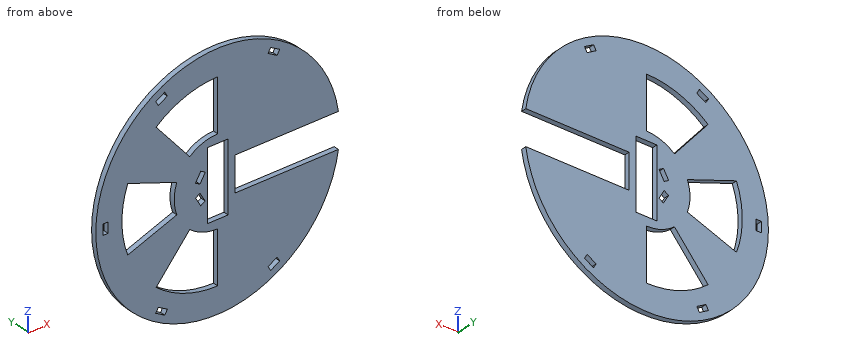
Autodesk Inventor part; units mm, degrees
ref_plane "YZ Plane" through (0, 0, 0) normal (1, 0, 0) x (0, 1, 0)
ref_plane "XZ Plane" through (0, 0, 0) normal (0, 1, 0) x (-1, 0, 0)
ref_plane "XY Plane" through (0, 0, 0) normal (0, 0, 1) x (1, 0, 0)
sketch "草圖1" plane through (0, 0, 0) normal (0, 1, 0) x (-1, 0, 0)
  circle A0 centre (0, 0) radius 70
  circle A1 centre (0, 0) radius 25
  line L0 (-70, 10) -> (-10, 10)
  line L1 (-10, 10) -> (-10, -10)
  line L2 (-10, -10) -> (-70, -10)
  line L3 (-70, -10) -> (-70, 10)
  line L4 (0, 0) -> (0, -55)
  line L5 (0, 0) -> (35.3533, -42.1324)
  arc A2 (0, -55) -> (35.3533, -42.1324) centre (0, 0) ccw
  line L6 (0, 0) -> (51.6831, -18.8111)
  line L7 (0, 0) -> (51.6831, 18.8111)
  arc A3 (51.6831, -18.8111) -> (51.6831, 18.8111) centre (0, 0) ccw
  line L8 (0, 0) -> (35.3533, 42.1324)
  line L9 (0, 0) -> (0, 55)
  arc A4 (35.3533, 42.1324) -> (0, 55) centre (0, 0) ccw
  line L10 (-9.3, -13.3795) -> (-36.7, -13.3795)
  line L11 (-36.7, -13.3795) -> (-36.7, -69.3795)
  line L12 (-36.7, -69.3795) -> (-9.3, -69.3795)
  line L13 (-9.3, -69.3795) -> (-9.3, -13.3795)
  line L14 (-7.8, -20.3795) -> (-10.8, -20.3795)
  line L15 (-10.8, -20.3795) -> (-10.8, -27.3795)
  line L16 (-10.8, -27.3795) -> (-7.8, -27.3795)
  line L17 (-7.8, -27.3795) -> (-7.8, -20.3795)
  line L18 (-7.8, -55.3795) -> (-10.8, -55.3795)
  line L19 (-10.8, -55.3795) -> (-10.8, -62.3795)
  line L20 (-10.8, -62.3795) -> (-7.8, -62.3795)
  line L21 (-7.8, -62.3795) -> (-7.8, -55.3795)
  line L22 (-35.2, -20.3795) -> (-38.2, -20.3795)
  line L23 (-38.2, -20.3795) -> (-38.2, -27.3795)
  line L24 (-38.2, -27.3795) -> (-35.2, -27.3795)
  line L25 (-35.2, -27.3795) -> (-35.2, -20.3795)
  line L26 (-35.2, -48.3795) -> (-38.2, -48.3795)
  line L27 (-38.2, -48.3795) -> (-38.2, -55.3795)
  line L28 (-38.2, -55.3795) -> (-35.2, -55.3795)
  line L29 (-35.2, -55.3795) -> (-35.2, -48.3795)
  circle A5 centre (0, 0) radius 2
  line L30 (-1.5, 1.3229) -> (-1.5, -1.3229)
  point P0 (-23, -13.3795)
  point P1 (-9.3, -20.3795)
  point P2 (-9.3, -62.3795)
  point P3 (-36.7, -20.3795)
  point P4 (-36.7, -48.3795)
  point P5 (16.0697, -19.1511)
  point P6 (0, -25)
  point P7 (-69.282, 10)
  point P8 (-69.282, -10)
  point P9 (16.0697, 19.1511)
  point P10 (0, 25)
  point P11 (23.4923, -8.5505)
  point P12 (23.4923, 8.5505)
  point P13 (-70, 0)
  dimension "d0" = 140
  dimension "d1" = 50
  dimension "d2" = 20
  dimension "d3" = 60
  dimension "d4" = 55
  dimension "d5" = 40
  dimension "d6" = 55
  dimension "d9" = 140
  dimension "d11" = 13
  dimension "d12" = 27.4
  dimension "d13" = 56
  dimension "d14" = 7
  dimension "d15" = 3
  dimension "d16" = 7
  dimension "d17" = 7
  dimension "d18" = 3
  dimension "d19" = 7
  dimension "d20" = 7
  dimension "d21" = 3
  dimension "d22" = 7
  dimension "d23" = 7
  dimension "d24" = 3
  dimension "d25" = 21
  dimension "d28" = 4
  dimension "d29" = 1.5
extrude "擠出1" add sketch "草圖1" along normal blind 3 contours L13 L20 L21 L18 L16 L17 A1 L4 A2 L5 L6 A3 L7 L8 A4 L9 L0 A0 | A0 L11 L28 L29 L26 L24 L25 L22 L10 A1 L15 L16 L13 L18 L19 L20 | A0 L2 A1 L10 L11 L22 L23 L24 L26 L27 L28 | L20 L19 L18 L13 | L13 L18 L21 L20 | L28 L27 L26 L11 | L11 L26 L29 L28 | A1 L9 A5 L4 L17 L14 L13 L10 L2 L1 L0 | L16 L15 A1 L13 | L13 A1 L17 L16 | A1 L8 A5 L9 | L10 L13 L14 L15 A1 | L24 L23 L22 L11 | L11 L22 L25 L24 | L13 L14 L17 A1 | A1 L15 L14 L13 | A1 L7 A5 L8 | A1 L6 A5 L7 | L30 A5 | L4 A5 L5 A1 | A5 L6 A1 L5
sketch "草圖2" plane through (0, 3, 0) normal (0, 1, 0) x (1, 0, 0)
  line L0 (-3, 13) -> (3, 13)
  line L1 (3, 13) -> (3, 10)
  line L2 (3, 10) -> (-3, 10)
  line L3 (-3, 10) -> (-3, 13)
  line L4 (-12.7583, 3.9019) -> (-9.7583, 9.0981)
  line L5 (-9.7583, 9.0981) -> (-7.1603, 7.5981)
  line L6 (-7.1603, 7.5981) -> (-10.1603, 2.4019)
  line L7 (-10.1603, 2.4019) -> (-12.7583, 3.9019)
  line L8 (-9.7583, -9.0981) -> (-12.7583, -3.9019)
  line L9 (-12.7583, -3.9019) -> (-10.1603, -2.4019)
  line L10 (-10.1603, -2.4019) -> (-7.1603, -7.5981)
  line L11 (-7.1603, -7.5981) -> (-9.7583, -9.0981)
  line L12 (3, -13) -> (-3, -13)
  line L13 (-3, -13) -> (-3, -10)
  line L14 (-3, -10) -> (3, -10)
  line L15 (3, -10) -> (3, -13)
  line L16 (-66, 3) -> (-63, 3)
  line L17 (-63, 3) -> (-63, -3)
  line L18 (-63, -3) -> (-66, -3)
  line L19 (-66, -3) -> (-66, 3)
  line L20 (-34.0981, -53.0596) -> (-28.9019, -56.0596)
  line L21 (-28.9019, -56.0596) -> (-30.4019, -58.6577)
  line L22 (-30.4019, -58.6577) -> (-35.5981, -55.6577)
  line L23 (-35.5981, -55.6577) -> (-34.0981, -53.0596)
  line L24 (28.9019, -56.0596) -> (34.0981, -53.0596)
  line L25 (34.0981, -53.0596) -> (35.5981, -55.6577)
  line L26 (35.5981, -55.6577) -> (30.4019, -58.6577)
  line L27 (30.4019, -58.6577) -> (28.9019, -56.0596)
  line L28 (63, -3) -> (63, 3)
  line L29 (63, 3) -> (66, 3)
  line L30 (66, 3) -> (66, -3)
  line L31 (66, -3) -> (63, -3)
  line L32 (34.0981, 53.0596) -> (28.9019, 56.0596)
  line L33 (28.9019, 56.0596) -> (30.4019, 58.6577)
  line L34 (30.4019, 58.6577) -> (35.5981, 55.6577)
  line L35 (35.5981, 55.6577) -> (34.0981, 53.0596)
  line L36 (-28.9019, 56.0596) -> (-34.0981, 53.0596)
  line L37 (-34.0981, 53.0596) -> (-35.5981, 55.6577)
  line L38 (-35.5981, 55.6577) -> (-30.4019, 58.6577)
  line L39 (-30.4019, 58.6577) -> (-28.9019, 56.0596)
  point P0 (0, 0)
  point P1 (0, 10)
  point P2 (-8.6603, 5)
  point P3 (-8.6603, -5)
  point P4 (0, -10)
  point P5 (-63, 0)
  point P6 (-31.5, -54.5596)
  point P7 (31.5, -54.5596)
  point P8 (63, 0)
  point P9 (31.5, 54.5596)
  point P10 (-31.5, 54.5596)
  dimension "d30" = 3
  dimension "d31" = 6
  dimension "d32" = 10
  dimension "d35" = 180
  dimension "d46" = 3
  dimension "d47" = 6
  dimension "d48" = 63
  dimension "d51" = 360
extrude "擠出2" cut sketch "草圖2" against normal through all contours L0 L1 L2 L3 | L4 L5 L6 L7 | L8 L9 L10 L11 | L12 L13 L14 L15 | L16 L17 L18 L19 | L20 L21 L22 L23 | L24 L25 L26 L27 | L32 L33 L34 L35 | L36 L37 L38 L39
sketch "草圖3" plane through (0, 3, 0) normal (0, 1, 0) x (1, 0, 0)
  circle A0 centre (0, 0) radius 6
  line L0 (-6, 20) -> (6, 20)
  line L1 (6, 20) -> (6, -20)
  line L2 (6, -20) -> (-6, -20)
  line L3 (-6, -20) -> (-6, 20)
  point P0 (6, 0)
  point P1 (0, 20)
  dimension "d53" = 12
  dimension "d54" = 40
  dimension "d55" = 12
extrude "擠出3" cut sketch "草圖3" against normal blind 10
properties material "MDF Medium Density Fiberboard"
For this review, take the finished solid that the model builds, in its own axes (mm). Coordinates: 2 decimals unless noted, no trailing zeros. Order: outer loops, then holes, each group sorted by start corner. A loop starts at its lowest first (then second) coordinate and runs counter-clockwise, first axis right, second up. Notation, with made-up numbers: (49, 7.5) -> (55, 7.5) arc R28 ccw to (55, 37.5) -> close; hole circle Ø6 at (-11.75, -16). An arc over 180 degrees is marked (long way). Return JSON: item names as keys, results as strings.
1. We need section A-A on z = 0. Write out the cut boundary in (x, y).
Answer block:
{"outline": "(-70, 0) -> (-66, 0) -> (-66, 3) -> (-70, 3) -> close; (-63, 0) -> (-55, 0) -> (-55, 3) -> (-63, 3) -> close; (-25, 0) -> (-6, 0) -> (-6, 3) -> (-25, 3) -> close; (6, 0) -> (10, 0) -> (10, 3) -> (6, 3) -> close"}
2. For pin 1 Ø1.5 at (x, y) = (-14.5, 0.5) entering from +Z; pin 2 Ø0.9 at (x, y) = (2.5, 2) entering from -Z; pin 3 Ø1.5 at (x, y) = (-65, 1) entering from -Z, all flat-tipped, find the tip position at first contact; note any pin that passes through.
Answer block:
{"pin 1": "z = 68.64", "pin 2": "z = -69.97", "pin 3": "z = -27.78"}
3. We need section D-D on z = 15. Write out the cut boundary in (x, y).
Answer block:
{"outline": "(-68.37, 0) -> (-52.92, 0) -> (-52.92, 3) -> (-68.37, 3) -> close; (-41.21, 0) -> (-6, 0) -> (-6, 3) -> (-41.21, 3) -> close; (6, 0) -> (68.37, 0) -> (68.37, 3) -> (6, 3) -> close"}
4. For line 1 (Z direction, x = 32.5, y = 1.75); line 2 (X direction, y = 1.3, z = 58.5); line 3 (X direction, y = 0.2, z = -1.5), list the stretches that pass through material, from the lowest coordinate up. Write a range as from..to.
Answer block:
{"line 1": "-62..-57.45, -53.98..-10, 10..53.98, 57.45..62", "line 2": "-38.44..-30.68, -30.31..30.31, 30.68..38.44", "line 3": "-69.98..-66, -63..-54.98, -24.95..-6, 6..10"}
5. We need section C-C on z = 50.5. Write out the cut boundary in (x, y).
Answer block:
{"outline": "(-48.47, 0) -> (-21.79, 0) -> (-21.79, 3) -> (-48.47, 3) -> close; (0, 0) -> (48.47, 0) -> (48.47, 3) -> (0, 3) -> close"}
6. We need section B-B on x = 59. Write out the cut boundary in (y, z).
Answer block:
{"outline": "(0, -37.67) -> (3, -37.67) -> (3, -10) -> (0, -10) -> close; (0, 10) -> (3, 10) -> (3, 37.67) -> (0, 37.67) -> close"}
